from build123d import *

# Parameters (mm, degrees)
SCHIZZO1_W                   = 449
SCHIZZO1_H                   = 94
SCHIZZO1_R                   = 7.8
SCHIZZO1_R_2                 = 2
ESTRUSIONE_ESTRUSIONE1_DEPTH = 4


with BuildPart() as part:
    # Schizzo1 → Estrusione-Estrusione1 (new body)
    with BuildSketch(Plane.XY):
        with Locations((-224.5, 47)):
            Rectangle(SCHIZZO1_W, SCHIZZO1_H)
        with Locations(Location((-384, 27, 0), (0, 0, 180))):
            Circle(SCHIZZO1_R, mode=Mode.SUBTRACT)
        with Locations((-9, 47)):
            Circle(SCHIZZO1_R_2, mode=Mode.SUBTRACT)
        with Locations((-224.5, 85)):
            Circle(SCHIZZO1_R_2, mode=Mode.SUBTRACT)
        with Locations(Location((-440, 47, 0), (0, 0, 180))):
            Circle(SCHIZZO1_R_2, mode=Mode.SUBTRACT)
        with Locations(Location((-224.5, 9, 0), (0, 0, 180))):
            Circle(SCHIZZO1_R_2, mode=Mode.SUBTRACT)
        with Locations((-324, 27)):
            Circle(SCHIZZO1_R, mode=Mode.SUBTRACT)
        with Locations(Location((-324, 67, 0), (0, 0, 180))):
            Circle(SCHIZZO1_R, mode=Mode.SUBTRACT)
        with Locations((-336.75, 85)):
            Circle(SCHIZZO1_R_2, mode=Mode.SUBTRACT)
        with Locations((-384, 67)):
            Circle(SCHIZZO1_R, mode=Mode.SUBTRACT)
        with Locations(Location((-336.75, 9, 0), (0, 0, 180))):
            Circle(SCHIZZO1_R_2, mode=Mode.SUBTRACT)
        with Locations((-112.25, 9)):
            Circle(SCHIZZO1_R_2, mode=Mode.SUBTRACT)
        with Locations(Location((-112.25, 85, 0), (0, 0, 180))):
            Circle(SCHIZZO1_R_2, mode=Mode.SUBTRACT)
        with Locations((-65, 67)):
            Circle(SCHIZZO1_R, mode=Mode.SUBTRACT)
        with Locations((-65, 27)):
            Circle(SCHIZZO1_R, mode=Mode.SUBTRACT)
        with Locations(Location((-125, 27, 0), (0, 0, 180))):
            Circle(SCHIZZO1_R, mode=Mode.SUBTRACT)
        with Locations(Location((-125, 67, 0), (0, 0, 180))):
            Circle(SCHIZZO1_R, mode=Mode.SUBTRACT)
    extrude(amount=ESTRUSIONE_ESTRUSIONE1_DEPTH)


solid = part.part
Read the model definition and answer for the solid it produces. Units are mm, in the model's axes. Give positions to 0.01 mm unless a question says otherwise; leave off trailing zeros. Loops run counter-clockwise (first coordinate to the right, second up) from the corner with the lowest first, then second, coordinate; pieces in that order, holes last. Notation, with made-up numbers: (39, -28.75) -> (97, -28.75) arc R15 cw to (97, -18.75) -> close; hole circle Ø1 at (-10, 0). An arc over 180 degrees is marked (long way). Answer as CSV lines item,"result".
Item 1: Find section C-C on z = 1.4. State how many separate pieces and enclosed holes the cut face has, plus the area to 3 significant figures.
Returned:
separate pieces,"1"
enclosed holes,"16"
area,"40,600 mm²"
Item 2: Find section A-A on x = -324. Give the vertices of the cut face in (y, z).
Returned:
outline,"(0, 0) -> (19.2, 0) -> (19.2, 4) -> (0, 4) -> close; (34.8, 0) -> (59.2, 0) -> (59.2, 4) -> (34.8, 4) -> close; (74.8, 0) -> (94, 0) -> (94, 4) -> (74.8, 4) -> close"
Item 3: Find section D-D on x = -387.5. Give the vertices of the cut face in (y, z).
Returned:
outline,"(0, 0) -> (20.03, 0) -> (20.03, 4) -> (0, 4) -> close; (33.97, 0) -> (60.03, 0) -> (60.03, 4) -> (33.97, 4) -> close; (73.97, 0) -> (94, 0) -> (94, 4) -> (73.97, 4) -> close"
Item 4: Determine the mould class of faces 1 (the face through (-228, 48, 4)), 2 (the face through (-72.792, 67.343, 1.972)) for opening direction Y: +Y half, -Y half, draft (parallel to the pull), parting line (faces both ways), or undercut.
Returned:
face 1,"draft"
face 2,"undercut"
Item 5: Consider line 1 (Y direction, x = -323.5, z = 3.6); line 2 (Y direction, x = -224.5, z = 2.15); line 3 (X direction, y = 30, z = 2.9). Determine where each line is inside the solid, lowest interval first. Write a range as [from, to].
Returned:
line 1,"y = [0, 19.22], [34.78, 59.22], [74.78, 94]"
line 2,"y = [0, 7], [11, 83], [87, 94]"
line 3,"x = [-449, -391.2], [-376.8, -331.2], [-316.8, -132.2], [-117.8, -72.2], [-57.8, 0]"
Item 6: Find section B-B on y = 27. Give the vertices of the cut face in (x, z), plus the area to 3 significant figures.
Returned:
outline,"(-449, 0) -> (-391.8, 0) -> (-391.8, 4) -> (-449, 4) -> close; (-376.2, 0) -> (-331.8, 0) -> (-331.8, 4) -> (-376.2, 4) -> close; (-316.2, 0) -> (-132.8, 0) -> (-132.8, 4) -> (-316.2, 4) -> close; (-117.2, 0) -> (-72.8, 0) -> (-72.8, 4) -> (-117.2, 4) -> close; (-57.2, 0) -> (0, 0) -> (0, 4) -> (-57.2, 4) -> close"
area,"1,550 mm²"
